Input: part model. Units: mm. Frame: model coordinates. Coordinates: 2 decimals unless noted, no trailing zeros. Loops run counter-clockwise (first coordinate to the right, second up) from the corner with the lowest first, then second, coordinate; pieces in that order, holes last.
(1) Section A-A, the plane x = -220. Return loops of the section in (y, z), then the cut area to 3 significant figures.
(2) Mould query, pull axis Z, two halves, no side actions, for faces 1 (the face through (-96, -47, 35.042)), 2 (the face through (-151, -53, 127.117)), 3 (the face through (-123.301, -46.958, 114.195)). Classes: released by +Z, released by -Z, zero draft, split by the parting line, or undercut.
(3) Line query: L1, parallel to Z at x = -146, y = -44.5; L2, parallel to Z at x = -112, y = -22.5; L3, parallel to X at y = -85, z = 52. Output: solid intervals per line, ascending.
(4) Contact query for flat-ended pins moving along their axis: P1, Ø5, axis at x = -99, y = -42, coming from the -Z side; P2, Ø18.5, axis at x = -214.5, y = -66.5, coming from the +Z side; P3, Ø12, axis at x = -93.5, y = -51, coming from the +Z side. Output: stop coordinate, or through.
(5) Section D-D, the plane x = -140. Return loops of the section in (y, z), then the cut area to 3 significant figures.
(6) Section C-C, the plane z = 46.5. Return loops of the section in (x, y).
(7) Section B-B, the plane y = -62. Give the number of separate pieces and of enclosed holes in the cut face, then the cut area to 3 significant figures.
```python
from build123d import *

# Parameters (mm, degrees)
F1_DEPTH = 12.7
F2_DEPTH = 95.25


# Not quite as in the source:
# - a feature names something its author has since deleted; it is built from what else it names


with BuildPart() as f1:
    # F0 (on Front) → F1 (new body)
    with BuildSketch(Plane.XZ):
        Polygon((-132.5943648094, 3.2924993012), (-114.2634937626, 35.0424993012), (-132.5943648094, 66.7924993012), (-169.2561069029, 66.7924993012), (-187.5869779497, 35.0424993012), (-169.2561069029, 3.2924993012), align=None)
        Polygon((-167.4230197982, 6.4674993012), (-183.9208037403, 35.0424993012), (-167.4230197982, 63.6174993012), (-134.427451914, 63.6174993012), (-117.929667972, 35.0424993012), (-134.427451914, 6.4674993012), align=None, mode=Mode.SUBTRACT)
        Polygon((-114.2634937626, 35.0424993012), (-77.6017516691, 35.0424993012), (-59.2708806223, 66.7924993012), (-77.6017516691, 98.5424993012), (-114.2634937626, 98.5424993012), (-132.5943648094, 66.7924993012), align=None)
        Polygon((-112.4304066579, 38.2174993012), (-128.9281906, 66.7924993012), (-112.4304066579, 95.3674993012), (-79.4348387737, 95.3674993012), (-62.9370548316, 66.7924993012), (-79.4348387737, 38.2174993012), align=None, mode=Mode.SUBTRACT)
        Polygon((-169.2561069029, 66.7924993012), (-132.5943648094, 66.7924993012), (-114.2634937626, 98.5424993012), (-132.5943648094, 130.2924993012), (-169.2561069029, 130.2924993012), (-187.5869779497, 98.5424993012), align=None)
        Polygon((-167.4230197982, 69.9674993012), (-183.9208037403, 98.5424993012), (-167.4230197982, 127.1174993012), (-134.427451914, 127.1174993012), (-117.929667972, 98.5424993012), (-134.427451914, 69.9674993012), align=None, mode=Mode.SUBTRACT)
        Polygon((-187.5869779497, 35.0424993012), (-169.2561069029, 66.7924993012), (-187.5869779497, 98.5424993012), (-190.6410588775, 98.5424993012), (-224.2487200432, 98.5424993012), (-242.57959109, 66.7924993012), (-224.2487200432, 35.0424993012), (-221.8035396555, 35.0424993012), align=None)
        Polygon((-222.4156329385, 38.2174993012), (-238.9134168806, 66.7924993012), (-222.4156329385, 95.3674993012), (-189.4200650544, 95.3674993012), (-172.9222811123, 66.7924993012), (-189.4200650544, 38.2174993012), align=None, mode=Mode.SUBTRACT)
        Polygon((-222.4156329385, 95.3674993012), (-238.9134168806, 66.7924993012), (-222.4156329385, 38.2174993012), (-189.4200650544, 38.2174993012), (-172.9222811123, 66.7924993012), (-189.4200650544, 95.3674993012), align=None)
        Polygon((-167.4230197982, 127.1174993012), (-183.9208037403, 98.5424993012), (-167.4230197982, 69.9674993012), (-134.427451914, 69.9674993012), (-117.929667972, 98.5424993012), (-134.427451914, 127.1174993012), align=None)
        Polygon((-167.4230197982, 63.6174993012), (-183.9208037403, 35.0424993012), (-167.4230197982, 6.4674993012), (-134.427451914, 6.4674993012), (-117.929667972, 35.0424993012), (-134.427451914, 63.6174993012), align=None)
        Polygon((-112.4304066579, 95.3674993012), (-128.9281906, 66.7924993012), (-112.4304066579, 38.2174993012), (-79.4348387737, 38.2174993012), (-62.9370548316, 66.7924993012), (-79.4348387737, 95.3674993012), align=None)
    extrude(amount=F1_DEPTH)

    # F0 (on Front) → F2 (join)
    with BuildSketch(Plane.XZ):
        Polygon((-114.2634937626, 35.0424993012), (-77.6017516691, 35.0424993012), (-59.2708806223, 66.7924993012), (-77.6017516691, 98.5424993012), (-114.2634937626, 98.5424993012), (-132.5943648094, 66.7924993012), align=None)
        Polygon((-112.4304066579, 38.2174993012), (-128.9281906, 66.7924993012), (-112.4304066579, 95.3674993012), (-79.4348387737, 95.3674993012), (-62.9370548316, 66.7924993012), (-79.4348387737, 38.2174993012), align=None, mode=Mode.SUBTRACT)
        Polygon((-77.6017516691, 98.5424993012), (-59.2708806223, 66.7924993012), (-57.4377935176, 69.9674993012), (-73.9355774597, 98.5424993012), align=None)
        Polygon((-132.5943648094, 3.2924993012), (-114.2634937626, 35.0424993012), (-132.5943648094, 66.7924993012), (-169.2561069029, 66.7924993012), (-187.5869779497, 35.0424993012), (-169.2561069029, 3.2924993012), align=None)
        Polygon((-167.4230197982, 6.4674993012), (-183.9208037403, 35.0424993012), (-167.4230197982, 63.6174993012), (-134.427451914, 63.6174993012), (-117.929667972, 35.0424993012), (-134.427451914, 6.4674993012), align=None, mode=Mode.SUBTRACT)
        Polygon((-169.2561069029, 66.7924993012), (-132.5943648094, 66.7924993012), (-114.2634937626, 98.5424993012), (-132.5943648094, 130.2924993012), (-169.2561069029, 130.2924993012), (-187.5869779497, 98.5424993012), align=None)
        Polygon((-167.4230197982, 69.9674993012), (-183.9208037403, 98.5424993012), (-167.4230197982, 127.1174993012), (-134.427451914, 127.1174993012), (-117.929667972, 98.5424993012), (-134.427451914, 69.9674993012), align=None, mode=Mode.SUBTRACT)
        Polygon((-172.9222811123, 3.2924993012), (-169.2561069029, 3.2924993012), (-187.5869779497, 35.0424993012), (-221.8035396555, 35.0424993012), (-224.2487200432, 35.0424993012), (-242.57959109, 66.7924993012), (-224.2487200432, 98.5424993012), (-190.6410588775, 98.5424993012), (-187.5869779497, 98.5424993012), (-169.2561069029, 130.2924993012), (-172.9222811123, 130.2924993011), (-189.4200650544, 101.7174993012), (-226.0818071479, 101.7174993012), (-246.2457652993, 66.7924993012), (-226.0818071479, 31.8674993012), (-189.4200650544, 31.8674993012), align=None)
        Polygon((-187.5869779497, 35.0424993012), (-169.2561069029, 66.7924993012), (-187.5869779497, 98.5424993012), (-190.6410588775, 98.5424993012), (-224.2487200432, 98.5424993012), (-242.57959109, 66.7924993012), (-224.2487200432, 35.0424993012), (-221.8035396555, 35.0424993012), align=None)
        Polygon((-222.4156329385, 38.2174993012), (-238.9134168806, 66.7924993012), (-222.4156329385, 95.3674993012), (-189.4200650544, 95.3674993012), (-172.9222811123, 66.7924993012), (-189.4200650544, 38.2174993012), align=None, mode=Mode.SUBTRACT)
    extrude(amount=F2_DEPTH)


solid = f1.part
```
Report:
1. outline: (-95.25, 31.87) - (0, 31.87) - (0, 101.72) - (-95.25, 101.72) - (-95.25, 95.37) - (-12.7, 95.37) - (-12.7, 38.22) - (-95.25, 38.22) - close
1. area: 1,940 mm2
2. face 1: released by -Z
2. face 2: undercut
2. face 3: released by +Z
3. L1: z = 3.29 to 6.47, 63.62 to 69.97, 127.12 to 130.29
3. L2: z = 35.04 to 38.22, 95.37 to 98.54
3. L3: x = -237.71 to -230.37, -181.46 to -174.13, -127.72 to -120.39, -71.48 to -67.81
4. P1: stops at z = 35.04
4. P2: stops at z = 101.72
4. P3: stops at z = 98.54
5. outline: (-95.25, 3.29) - (0, 3.29) - (0, 130.29) - (-95.25, 130.29) - (-95.25, 127.12) - (-12.7, 127.12) - (-12.7, 69.97) - (-95.25, 69.97) - (-95.25, 63.62) - (-12.7, 63.62) - (-12.7, 6.47) - (-95.25, 6.47) - close
5. area: 2,660 mm2
6. outline: (-234.53, -95.25) - (-227.2, -95.25) - (-227.2, -12.7) - (-184.64, -12.7) - (-184.64, -95.25) - (-177.31, -95.25) - (-177.31, -12.7) - (-124.54, -12.7) - (-124.54, -95.25) - (-117.21, -95.25) - (-117.21, -12.7) - (-74.65, -12.7) - (-74.65, -95.25) - (-70.99, -95.25) - (-70.99, 0) - (-234.53, 0) - close
7. separate pieces: 1
7. enclosed holes: 4
7. area: 3,460 mm2
